The listing builds one solid part. Answer for the finished solid, in the listing's coordinates (mm). Face numbers are marked on the shaded views. A direction names the side the tool comes from. Round coordinates to 2 decimals unless told otherwise and drop trailing zeros. Loops run counter-clockwise (first coordinate to the right, second up) from the corner with the lowest first, then second, coordinate; pieces in that order, holes last. Notation, with made-up numbers: M -16.75,59 L 12.25,59 A15 cw 12.25,63 Z; hole C 83,77.25 d8. An arc over 180 degrees is marked long. Put each result on its own line as item: value. Start each with the question number.
(1) Section D-D, the plane x = 0 is taken. Determine the outline of the cut face in (y, z) (3 decimals), then the cut area to 3 significant figures.
(2) Determine the mould class of the marked faces 1, 2 and 3 for opening direction X: released by +X, released by -X, zero draft, split by the parting line, or undercut.
(3) Section B-B, the plane x = 28 is taken. Determine the outline of the cut face in (y, z).
(4) Which of the six approach directions +Z, -Z, +X, -X, +Y, -Y give full straight-line access (tool end or side, diameter ignored) to the marked faces 4 and 5?
(5) Flat-ended cylindrical pins translate along their axes: P1, Ø4, axis at y = -25, z = 42.5, coming from the +X side; P2, Ø10, axis at y = -18, z = 27, coming from the +X side (3 decimals); P3, Ø1.9, axis at y = -23.5, z = 44, coming from the +X side. Find the tip coordinate at first contact, or state that the pin passes through.
(6) Section C-C, the plane z = 77 is taken. Determine the outline of the cut face in (x, y) (3 decimals).
(7) Straight lines are drawn through the part: line 1 (Y direction, x = 12, z = 24) (3 decimals); line 2 (Y direction, x = 0, z = 55) (3 decimals); line 3 (Y direction, x = 27, z = 5). For each, find the intervals that lie inside material, in ascending order.
(8) Section A-A, the plane y = 0 is taken. Determine the outline of the cut face in (x, z) (3 decimals), then the cut area to 3 significant figures.
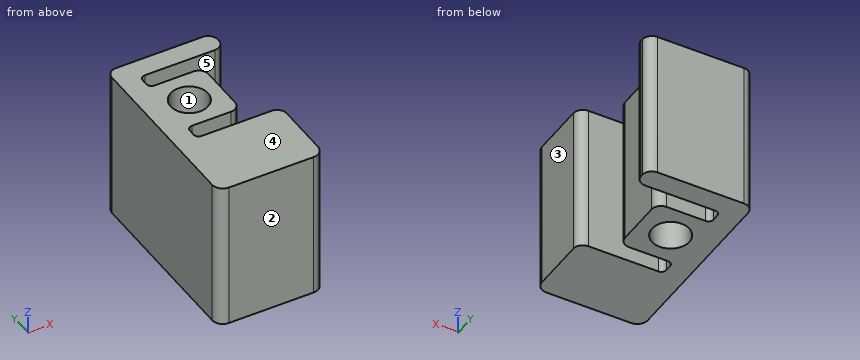
```python
from build123d import *

# Parameters (mm, degrees)
SKETCH1_R           = 11.2
BOSS_EXTRUDE1_DEPTH = 89.651758212


with BuildPart() as part:
    # Sketch1 → Boss-Extrude1 (new body)
    with BuildSketch(Plane.XY):
        with BuildLine():
            Line((-25.4, -67.479999962), (-25.4, 36.365))
            ThreePointArc((-25.4, 36.365), (-23.726115254, 40.406115254), (-19.685, 42.08))
            Line((-19.685, 42.08), (32.385, 42.08))
            ThreePointArc((32.385, 42.08), (36.426115254, 40.406115254), (38.1, 36.365))
            Line((38.1, 36.365), (38.1, 35.095))
            ThreePointArc((38.1, 35.095), (36.426115254, 31.053884746), (32.385, 29.38))
            Line((32.385, 29.38), (-9.652, 29.38))
            ThreePointArc((-9.652, 29.38), (-11.807261469, 28.487261469), (-12.7, 26.332))
            Line((-12.7, 26.332), (-12.7, 22.503))
            ThreePointArc((-12.7, 22.503), (-11.807261469, 20.347738531), (-9.652, 19.455))
            Line((-9.652, 19.455), (0, 19.455))
            Line((0, 19.455), (13.74, 19.455))
            ThreePointArc((13.74, 19.455), (17.781115254, 17.781115254), (19.455, 13.74))
            Line((19.455, 13.74), (19.455, 0))
            Line((19.455, 0), (19.455, -13.74))
            ThreePointArc((19.455, -13.74), (17.781115254, -17.781115254), (13.74, -19.455))
            Line((13.74, -19.455), (0, -19.455))
            Line((0, -19.455), (-9.652, -19.455))
            ThreePointArc((-9.652, -19.455), (-11.807261469, -20.347738531), (-12.7, -22.503))
            Line((-12.7, -22.503), (-12.7, -26.331999962))
            ThreePointArc((-12.7, -26.331999962), (-11.807261469, -28.487261431), (-9.652, -29.379999962))
            Line((-9.652, -29.379999962), (32.385, -29.379999962))
            ThreePointArc((32.385, -29.379999962), (36.426115254, -31.053884708), (38.1, -35.094999962))
            Line((38.1, -35.094999962), (38.1, -67.479999962))
            ThreePointArc((38.1, -67.479999962), (36.240128061, -71.970128023), (31.75, -73.829999962))
            Line((31.75, -73.829999962), (-19.05, -73.829999962))
            ThreePointArc((-19.05, -73.829999962), (-23.540128061, -71.970128023), (-25.4, -67.479999962))
        make_face()
        Circle(SKETCH1_R, mode=Mode.SUBTRACT)
    extrude(amount=BOSS_EXTRUDE1_DEPTH)


solid = part.part
```
Recorded:
1. outline: M -73.83,0 L -29.38,0 L -29.38,89.652 L -73.83,89.652 Z; M -19.455,0 L -11.2,0 L -11.2,89.652 L -19.455,89.652 Z; M 11.2,0 L 19.455,0 L 19.455,89.652 L 11.2,89.652 Z; M 29.38,0 L 42.08,0 L 42.08,89.652 L 29.38,89.652 Z
1. area: 6,600 mm²
2. face 1: undercut
2. face 2: zero draft
2. face 3: released by +X
3. outline: M -73.83,0 L -29.38,0 L -29.38,89.65 L -73.83,89.65 Z; M 29.38,0 L 42.08,0 L 42.08,89.65 L 29.38,89.65 Z
4. face 4: +Z, +X, -X, +Y, -Y
4. face 5: +Z, -Z, +X
5. P1: stops at x = -12.63
5. P2: stops at x = 19.455
5. P3: stops at x = -12.7
6. outline: M -25.4,-67.48 A6.35 ccw -19.05,-73.83 L 31.75,-73.83 A6.35 ccw 38.1,-67.48 L 38.1,-35.095 A5.715 ccw 32.385,-29.38 L -9.652,-29.38 A3.048 cw -12.7,-26.332 L -12.7,-22.503 A3.048 cw -9.652,-19.455 L 13.74,-19.455 A5.715 ccw 19.455,-13.74 L 19.455,13.74 A5.715 ccw 13.74,19.455 L -9.652,19.455 A3.048 cw -12.7,22.503 L -12.7,26.332 A3.048 cw -9.652,29.38 L 32.385,29.38 A5.715 ccw 38.1,35.095 L 38.1,36.365 A5.715 ccw 32.385,42.08 L -19.685,42.08 A5.715 ccw -25.4,36.365 Z; hole C 0,0 d22.4
7. line 1: y = -73.83 to -29.38, -19.455 to 19.455, 29.38 to 42.08
7. line 2: y = -73.83 to -29.38, -19.455 to -11.2, 11.2 to 19.455, 29.38 to 42.08
7. line 3: y = -73.83 to -29.38, 29.38 to 42.08
8. outline: M -25.4,0 L -11.2,0 L -11.2,89.652 L -25.4,89.652 Z; M 11.2,0 L 19.455,0 L 19.455,89.652 L 11.2,89.652 Z
8. area: 2,010 mm²
